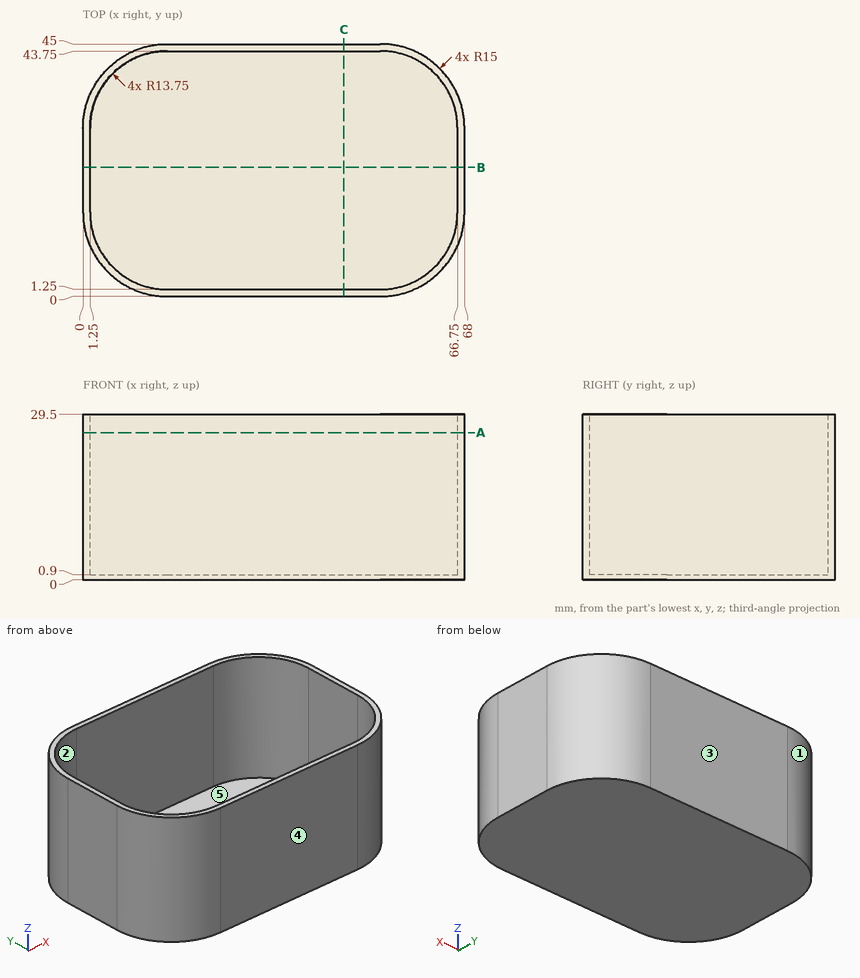
Source: three-view drawing plus pictorial views. Frame: mm from the lowest corner of the part. A direction names the side the tool comes from. Round coordinates to 2 decimals unless told otherwise and drop trailing zeros. Order: outer loops, then holes, each group sorted by start corner. A loop starts at its lowest first (then second) coordinate and runs counter-clockwise, first axis right, second up. Notation, with made-up numbers: (15, -37) -> (25, -37) arc R23 cw to (25, -3) -> close; hole circle Ø2 at (-23, -17.75). An arc over 180 degrees is marked (long way). Use one line per item in the form item = value.
(1) Access query for the marked faces 1 and 2. Directions: +Z, -Z, +X, -X, +Y, -Y. A direction counts if a zero-diameter tool reaches every point of the face in a straight line with its end or side. Return the directions, or none.
Results list:
face_1 = +Z, -Z, -X, +Y
face_2 = +Z
(2) Section A-A on z = 26.25. Return loops of the section in (x, y), and give its area (3 significant figures).
Results list:
outline = (0, 15) arc R15 ccw to (15, 0) -> (53, 0) arc R15 ccw to (68, 15) -> (68, 30) arc R15 ccw to (53, 45) -> (15, 45) arc R15 ccw to (0, 30) -> close; hole (1.25, 15) arc R13.75 ccw to (15, 1.25) -> (53, 1.25) arc R13.75 ccw to (66.75, 15) -> (66.75, 30) arc R13.75 ccw to (53, 43.75) -> (15, 43.75) arc R13.75 ccw to (1.25, 30) -> close
area = 245 mm^2
(3) First-contact query: pin 1 Ø5 at (y, z) = (39, 16.5) entering from -X; pin 2 Ø13 at (x, y) = (44, 18) entering from +Z; pin 3 Ø6 at (y, z) = (11.5, 3.5) entering from -X. Flat tips, straight axial feed; report the tip coordinate or a pass-through.
Results list:
pin_1 = 1.48
pin_2 = 0.9
pin_3 = 0.01
(4) Section B-B on y = 23. Return loops of the section in (x, z).
Results list:
outline = (0, 0) -> (68, 0) -> (68, 29.5) -> (66.75, 29.5) -> (66.75, 0.9) -> (1.25, 0.9) -> (1.25, 29.5) -> (0, 29.5) -> close
(5) Draft query along Y for the marked faces 3, 4 and 5. Return one class per face: pulls with the +Y half, pulls with the -Y half, needs draft (parallel to the pull), parting line crosses it, or undercut.
Results list:
face_3 = pulls with the +Y half
face_4 = pulls with the -Y half
face_5 = undercut
(6) Section C-C on x = 46.5. Return loops of the section in (y, z), and give its area (3 significant figures).
Results list:
outline = (0, 0) -> (45, 0) -> (45, 29.5) -> (43.75, 29.5) -> (43.75, 0.9) -> (1.25, 0.9) -> (1.25, 29.5) -> (0, 29.5) -> close
area = 112 mm^2
(7) Ray query, probe 1 along Y at (x, z) = (40, 6); probe 2 along X at (y, z) = (21, 16.75); probe 3 along X at (y, z) = (30.5, 8). Return the intervals inside material, ascending. Write a range as [from, to].
Results list:
probe_1 = [0, 1.25], [43.75, 45]
probe_2 = [0, 1.25], [66.75, 68]
probe_3 = [0.01, 1.26], [66.74, 67.99]
